```python
from build123d import *

# Parameters (mm, degrees)
SKETCH_1_R          = 1.4
SKETCH_1_R_2        = 1.65
EXTRUDE_1_DEPTH     = 3
SKETCH_2_R          = 0.6
CUT_EXTRUDE_1_DEPTH = 34.421549934
CHAMFER_2_SIZE      = 0.5
CHAMFER_3_SIZE      = 0.5


with BuildPart() as part:
    # 草图1 → 凸台-拉伸1 (new body)
    with BuildSketch(Plane.XY):
        Polygon((-8, 7), (-3.705865331, 4), (4.294134669, 4), (8, 7), (24, 7), (24, -11), (-28, -11), (-28, 7), align=None)
        with Locations((-18, 3)):
            Circle(SKETCH_1_R, mode=Mode.SUBTRACT)
        with Locations((4, -5.5)):
            Circle(SKETCH_1_R, mode=Mode.SUBTRACT)
        with Locations((-24, -8)):
            Circle(SKETCH_1_R_2, mode=Mode.SUBTRACT)
        with Locations((10, -8)):
            Circle(SKETCH_1_R_2, mode=Mode.SUBTRACT)
    extrude(amount=EXTRUDE_1_DEPTH)

    # 草图2 → 切除-拉伸1 (cut, through all)
    with BuildSketch(Plane.XZ.offset(11)):
        with Locations(Location((12.1, 1.5, 0), (0, 0, 270))):
            Circle(SKETCH_2_R)
        with Locations(Location((-12, 1.5, 0), (0, 0, 270))):
            Circle(SKETCH_2_R)
    extrude(amount=-CUT_EXTRUDE_1_DEPTH, mode=Mode.SUBTRACT)

    # 倒角2
    chamfer_2_edges = [part.edges().sort_by_distance(p)[0] for p in [
        (24, -2, 0),
        (24, -11, 1.5),
        (-28, -11, 1.5),
        (-28, 7, 1.5),
        (24, 7, 1.5),
        (-28, -2, 3),
        (24, -2, 3),
        (-28, -2, 0),
    ]]
    chamfer(chamfer_2_edges, length=CHAMFER_2_SIZE)

    # 倒角3
    chamfer_3_edges = [part.edges().sort_by_distance(p)[0] for p in [
        (0.294134669, 4, 0),
        (6.147067334, 5.5, 0),
        (6.147067334, 5.5, 3),
        (0.294134669, 4, 3),
        (-5.852932666, 5.5, 3),
        (-17.75, 7, 3),
        (15.75, 7, 3),
        (-2, -11, 3),
        (-2, -11, 0),
        (15.75, 7, 0),
        (-17.75, 7, 0),
        (-5.852932666, 5.5, 0),
    ]]
    chamfer(chamfer_3_edges, length=CHAMFER_3_SIZE)


solid = part.part
```
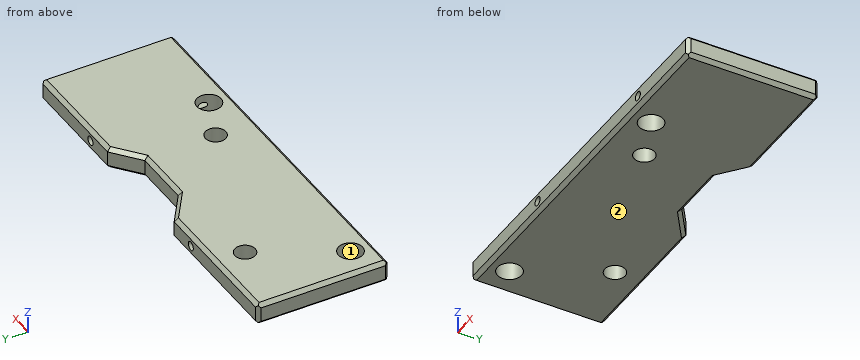
Could you check a few things on this model? Use its own coordinates, in mm. Face numbers are marked on the shaded views. Give positions to 0.01 mm unless a question says otherwise; leave off trailing zeros. Order: outer loops, then holes, each group sorted by start corner. A loop starts at its lowest first (then second) coordinate and runs counter-clockwise, first axis right, second up.
Q1. Suppose I cut it at A-A, the plane y = 3. Write out the boundary of the cut face in (x, z).
Q2. We'd pull the mould along Y, two halves only. Please class the marked faces 1 and 2: +Y half, -Y half, draft (parallel to the pull), parting line (faces both ways), or undercut.
Q3. Suppose I cut it at B-B, the plane y = -8. Write out the boundary of the cut face in (x, z).
Q4. Suppose I cut it at D-D, the plane x = -6.5. Write out the boundary of the cut face in (y, z), and give its area (3 significant figures).
Q5. I'm going to push a flat-ended pin straight in: P1, Ø0.6, axis at x = -1, z = 2, coming from the +Y side. Where does the tip first touch, or does it pass through?
Q6. If I drill on line 1 along X through (y, z) = (1, 1.5); line 2 along X through (y, z) = (-10, 2); line 3 along X through (y, z) = (-4.25, 1.5), over which ranges is the centre line in solid material (lowest first)?
Q7. Suppose I cut it at C-C, the plane x = 12.1. Write out the boundary of the cut face in (y, z).
Solution:
1. outline: (-28, 0.5) - (-27.5, 0) - (-19.4, 0) - (-19.4, 3) - (-27.5, 3) - (-28, 2.5) - close; (-16.6, 0) - (23.5, 0) - (24, 0.5) - (24, 2.5) - (23.5, 3) - (-16.6, 3) - close; hole circle Ø1.2 at (-12, 1.5); hole circle Ø1.2 at (12.1, 1.5)
2. face 1: undercut
2. face 2: draft
3. outline: (-28, 0.5) - (-27.5, 0) - (-25.65, 0) - (-25.65, 3) - (-27.5, 3) - (-28, 2.5) - close; (-22.35, 0) - (8.35, 0) - (8.35, 3) - (-22.35, 3) - close; (11.65, 0) - (23.5, 0) - (24, 0.5) - (24, 2.5) - (23.5, 3) - (11.65, 3) - (11.65, 1.9) arc R0.6 cw (long way) to (11.65, 1.1) - close; hole circle Ø1.2 at (-12, 1.5)
4. outline: (-11, 0.5) - (-10.5, 0) - (5.34, 0) - (5.95, 0.5) - (5.95, 2.5) - (5.34, 3) - (-10.5, 3) - (-11, 2.5) - close
4. area: 50.3 mm2
5. P1: stops at y = 4
6. line 1: x = -28 to -12.6, -11.4 to 11.5, 12.7 to 24
6. line 2: x = -28 to -12.33, -11.67 to 11.77, 12.43 to 24
6. line 3: x = -28 to -12.6, -11.4 to 3.37, 4.63 to 11.5, 12.7 to 24
7. outline: (-11, 0.5) - (-10.5, 0) - (6.5, 0) - (7, 0.5) - (7, 0.9) - (-11, 0.9) - close; (-11, 2.1) - (7, 2.1) - (7, 2.5) - (6.5, 3) - (-10.5, 3) - (-11, 2.5) - close
